Print and shaded views of the part. All mm, measured from the part's lowest x, y and z. A direction names the side the tool comes from. Coordinates: 2 decimals unless noted, no trailing zeros. Loops run counter-clockwise (first coordinate to the right, second up) from the corner with the lowest first, then second, coordinate; pieces in that order, holes last. Notation, with made-up numbers: M 18.25,41.25 L 61.25,41.25 A14 ccw 61.25,59.25 Z; hole C 39.5,60.25 d10. An arc over 180 degrees is marked long. Use a Markdown table: item, result. Add a question column.
1) Band-saw the part on D-D (x = 22). List the corners of the cut face in (y, z), plus the area to 3 significant figures.
2) Tool access for the marked faces 4, 5, 6 and 7: list every direction of +Z, -Z, +X, -X, +Y, -Y with a clear straight run to the whole face (end or side of a thin tool).
3) Band-saw the part on B-B (y = 16). List the corners of the cut face in (x, z), plus the area to 3 significant figures.
4) Band-saw the part on A-A (x = 14). List the corners of the cut face in (y, z).
5) Pull direction X, two halves, no side cores. Call the marked faces 1, 2 and 3: released by +X, released by -X, zero draft, split by the parting line, or undercut.
6) Wall check: probe 1 along Y at (x, z) = (13.5, 11.75); probe 2 along Z at (x, y) = (22, 41.3); probe 3 along Z at (x, y) = (25.5, 18). Give the ranges that are in metal, low to high. Write a range as from..to.
7) Pin check, flat tips, straight feed: pin 1 Ø3 at (x, y) = (23.5, 8.5) entering from +Z; pin 2 Ø16 at (x, y) = (14, 16) entering from -Z; pin 3 Ø5 at (x, z) = (6, 5) entering from -Y; pin 4 Ø4 at (y, z) = (42, 27) entering from -X. Stop position of each tip, or through.
8) Band-saw the part on C-C (z = 19.5). List the corners of the cut face in (x, y), plus the area to 3 significant figures.
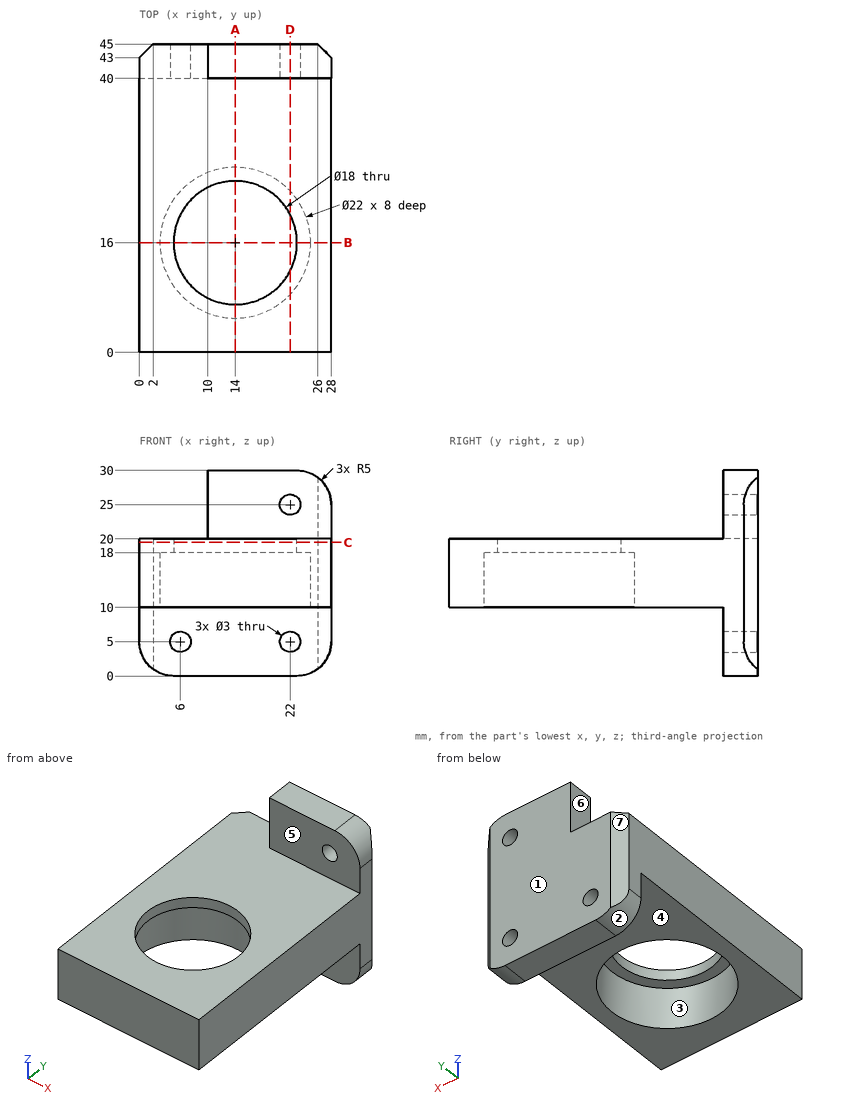
Entries:
| question | item | result |
|---|---|---|
| 1 | outline | M 0,10 L 8.45,10 L 8.45,18 L 11.88,18 L 11.88,20 L 0,20 Z; M 20.12,18 L 23.55,18 L 23.55,10 L 40,10 L 40,6.5 L 45,6.5 L 45,23.5 L 40,23.5 L 40,20 L 20.12,20 Z; M 40,0 L 45,0 L 45,3.5 L 40,3.5 Z; M 40,26.5 L 45,26.5 L 45,30 L 40,30 Z |
| 1 | area | 383 mm2 |
| 2 | face 4 | -Z, +X, -X, -Y |
| 2 | face 5 | +Z, +X, -X, -Y |
| 2 | face 6 | +Z, -X, +Y, -Y |
| 2 | face 7 | +Z, -Z, -X, +Y |
| 3 | outline | M 0,10 L 3,10 L 3,18 L 5,18 L 5,20 L 0,20 Z; M 23,18 L 25,18 L 25,10 L 28,10 L 28,20 L 23,20 Z |
| 3 | area | 68.0 mm2 |
| 4 | outline | M 0,10 L 5,10 L 5,18 L 7,18 L 7,20 L 0,20 Z; M 25,18 L 27,18 L 27,10 L 40,10 L 40,0 L 45,0 L 45,30 L 40,30 L 40,20 L 25,20 Z |
| 5 | face 1 | zero draft |
| 5 | face 2 | released by -X |
| 5 | face 3 | undercut |
| 6 | probe 1 | 0..5.01, 26.99..45 |
| 6 | probe 2 | 0..3.5, 6.5..23.5, 26.5..30 |
| 6 | probe 3 | 10..20 |
| 7 | pin 1 | z = 20 |
| 7 | pin 2 | through |
| 7 | pin 3 | y = 40 |
| 7 | pin 4 | x = 10 |
| 8 | outline | M 0,0 L 28,0 L 28,43 L 26,45 L 2,45 L 0,43 Z; hole C 14,16 d18 |
| 8 | area | 1,000 mm2 |
